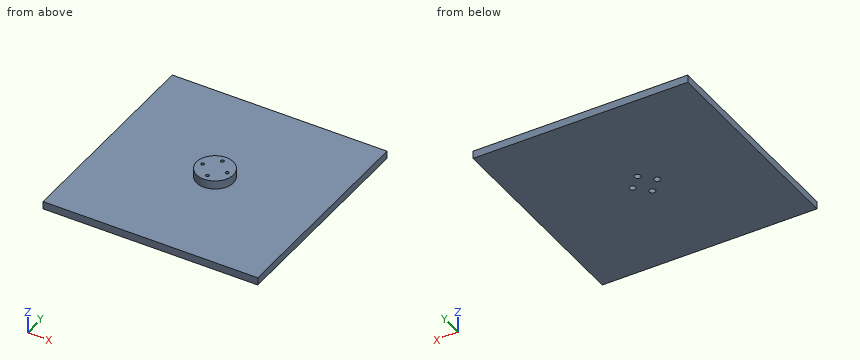
```python
from build123d import *

# Parameters (mm, degrees)
F0_W           = 140
F0_H           = 140
F0_R           = 12
F1_DEPTH       = 5
F2_DEPTH       = 10.56
F3_D           = 2.2
F3_DEPTH       = 12
F3_CBORE_D     = 4
F3_CBORE_DEPTH = 8
F3_TIP         = 0.6609466809


# Not quite as in the source:
# - a feature names something its author has since deleted; it is built from what else it names


with BuildPart() as f1:
    # F0 (on Top) → F1 (new body)
    with BuildSketch(Plane.XY):
        Rectangle(F0_W, F0_H)
        Circle(F0_R, mode=Mode.SUBTRACT)
    extrude(amount=F1_DEPTH)

    # F0 (on Top) → F2 (join)
    with BuildSketch(Plane.XY):
        Circle(F0_R)
    extrude(amount=F2_DEPTH)

    # F3
    with Locations(Plane(origin=(0, 0, 0), x_dir=(1, 0, 0), z_dir=(0, 0, -1))):
        with Locations((8, 0), (0, -8), (-8, 0), (0, 8)):
            CounterBoreHole(F3_D / 2, F3_CBORE_D / 2, F3_CBORE_DEPTH, depth=F3_DEPTH)
            with Locations((0, 0, -(F3_DEPTH + F3_TIP / 2))):  # 118° drill point
                Cone(0, F3_D / 2, F3_TIP, mode=Mode.SUBTRACT)


solid = f1.part
```
Model file for the job. Use its own axes, mm. Coordinates: 2 decimals unless noted, no trailing zeros. Loops run counter-clockwise (first coordinate to the right, second up) from the corner with the lowest first, then second, coordinate; pieces in that order, holes last. Notation, with made-up numbers: (74, -35) -> (101, -35) arc R33 ccw to (101, 3) -> close; hole circle Ø3 at (9, -1.75). An arc over 180 degrees is marked (long way). Answer as a JSON object with one key per item and string values.
Q1. Probe probe 1 along Y at (x, z) = (0, 3.25); probe 2 along Y at (x, z) = (0, 9); probe 3 along Z at (x, y) = (-31.5, -10). List the from-to ranges inside material, lowest first.
Report:
{"probe 1": "y = -70 to -10, -6 to 6, 10 to 70", "probe 2": "y = -12 to -9.1, -6.9 to 6.9, 9.1 to 12", "probe 3": "z = 0 to 5"}
Q2. Cut at A-A (y = 59.5). List the corners of the cut face in (x, z), and give its area (3 significant figures).
Report:
{"outline": "(-70, 0) -> (70, 0) -> (70, 5) -> (-70, 5) -> close", "area": "700 mm2"}
Q3. Flat gauge pins, fed straight in: P1, Ø3, axis at x = -22.5, y = 36.5, coming from the +Z side; P2, Ø3, axis at x = 8, y = 0, coming from the -Z side. Where does each tip first touch, or does it go through?
Report:
{"P1": "stops at z = 5", "P2": "stops at z = 8"}
